Here's how the part is built. I have some questions about the finished solid (model axes, mm). Face numbers are marked on the shaded views. A direction names the side the tool comes from. Round coordinates to 2 decimals unless told otherwise and drop trailing zeros. Loops run counter-clockwise (first coordinate to the right, second up) from the corner with the lowest first, then second, coordinate; pieces in that order, holes last. Notation, with made-up numbers: M 82,39 L 98,39 A23 ccw 98,52 Z; hole C -35.75,-23.5 d9. An arc over 180 degrees is marked long. Answer as CSV lines item,"result".
```python
from build123d import *

# Parameters (mm, degrees)
SKETCH1_R           = 1
SKETCH1_R_2         = 0.5
SKETCH1_R_3         = 1.75
BOSS_EXTRUDE1_DEPTH = 2
FILLET1_R           = 2


with BuildPart() as part:
    # Sketch1 → Boss-Extrude1 (new body)
    with BuildSketch(Plane(origin=(0, 0, 0), x_dir=(1, 0, 0), z_dir=(0, 1, 0))):
        Polygon((-12.864326531, 1.102455199), (6.635673469, 1.102455199), (6.635673469, -10.897544801), (-12.864326531, -10.897544801), (-12.864326531, -4.397544801), (-21.064326531, -4.397544801), (-21.064326531, 1.102455199), align=None)
        with Locations(Location((-9.864326531, -1.897544801, 0), (0, 0, 270))):
            Circle(SKETCH1_R, mode=Mode.SUBTRACT)
        with Locations(Location((3.635673469, -1.897544801, 0), (0, 0, 270))):
            Circle(SKETCH1_R, mode=Mode.SUBTRACT)
        with Locations(Location((-11.764326531, -8.897544801, 0), (0, 0, 270))):
            Circle(SKETCH1_R_2, mode=Mode.SUBTRACT)
        with Locations(Location((-1.764326531, -8.897544801, 0), (0, 0, 270))):
            Circle(SKETCH1_R_2, mode=Mode.SUBTRACT)
        with Locations(Location((-18.064326531, -1.397544801, 0), (0, 0, 270))):
            Circle(SKETCH1_R_3, mode=Mode.SUBTRACT)
    extrude(amount=BOSS_EXTRUDE1_DEPTH)

    # Fillet1
    fillet1_edges = [part.edges().sort_by_distance(p)[0] for p in [
        (6.635673469, 1, -1.102455199),
        (6.635673469, 1, 10.897544801),
        (-12.864326531, 1, 10.897544801),
        (-12.864326531, 1, 4.397544801),
        (-21.064326531, 1, 4.397544801),
        (-21.064326531, 1, -1.102455199),
    ]]
    fillet(fillet1_edges, radius=FILLET1_R)


solid = part.part
```
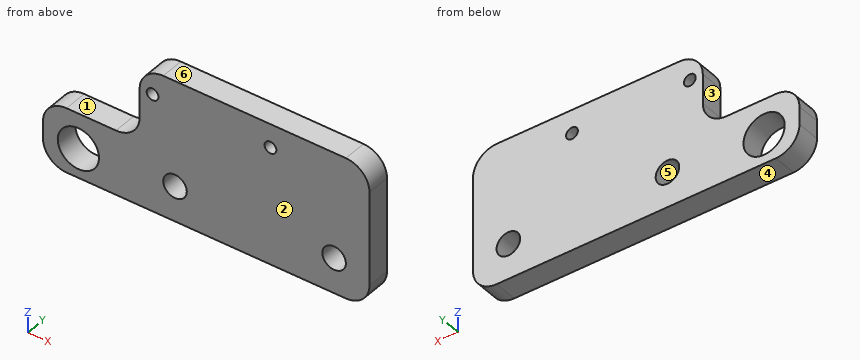
1. For P1, Ø0.6, axis at x = -16.5, y = 1, coming from the +Z side; P2, Ø1.6, axis at x = -9.86, z = 1.9, coming from the +Y side; P3, Ø1, axis at y = 1, z = 8, coming from the -X side, each with a flat end and sliding along its axis, tell me the tip position at first contact or that it passes through.
Evaluation:
P1,"stops at z = 4.4"
P2,"passes through"
P3,"stops at x = -12.86"
2. Which directions (+Z, -Z, +X, -X, +Y, -Y) give clear straight access to the entire face, cutting with the end or side of a thin tool? Please do the marked faces 1 and 2.
Evaluation:
face 1,"+Z, -X, +Y, -Y"
face 2,"+Z, -Z, +X, -X, -Y"
3. I want a section at B-B, the plane x = -18.75. Please give me the cut outline in (y, z).
Evaluation:
outline,"M 0,-1.1 L 2,-1.1 L 2,-0.21 L 0,-0.21 Z; M 0,3.01 L 2,3.01 L 2,4.4 L 0,4.4 Z"
4. If I drill on line 1 (X direction, y = 1.1, z = 8.75); line 2 (X direction, y = 0.25, z = 2.25); line 3 (X direction, y = 0.85, z = 2.5), over which ranges is the centre line in solid material (lowest first)? Write a range as [from, to].
Evaluation:
line 1,"x = [-12.86, -12.24], [-11.29, -2.24], [-1.29, 6.64]"
line 2,"x = [-21.06, -19.59], [-16.54, -10.8], [-8.93, 2.7], [4.57, 6.64]"
line 3,"x = [-21.06, -19.42], [-16.71, -10.66], [-9.07, 2.84], [4.43, 6.64]"
5. We'd pull the mould along Z, two halves only. Please class the marked faces 3, 4, 5 and 6: pulls with the +Z half, pulls with the -Z half, needs draft (parallel to the pull), parting line crosses it, or undercut.
Evaluation:
face 3,"needs draft"
face 4,"pulls with the -Z half"
face 5,"undercut"
face 6,"pulls with the +Z half"
6. I want a section at A-A, the plane y = 1.5. Please give me the cut outline in (x, z), and give its area (3 significant figures).
Evaluation:
outline,"M -21.06,0.9 A2 ccw -19.06,-1.1 L 4.64,-1.1 A2 ccw 6.64,0.9 L 6.64,8.9 A2 ccw 4.64,10.9 L -10.86,10.9 A2 ccw -12.86,8.9 L -12.86,6.4 A2 cw -14.86,4.4 L -19.06,4.4 A2 ccw -21.06,2.4 Z; hole C -18.06,1.4 d3.5; hole C -11.76,8.9 d1; hole C -9.86,1.9 d2; hole C -1.76,8.9 d1; hole C 3.64,1.9 d2"
area,"258 mm²"
7. I want a section at D-D, the plane z = 1.75. Please give me the cut outline in (x, y).
Evaluation:
outline,"M -21.06,0 L -19.78,0 L -19.78,2 L -21.06,2 Z; M -16.35,0 L -10.85,0 L -10.85,2 L -16.35,2 Z; M -8.88,0 L 2.65,0 L 2.65,2 L -8.88,2 Z; M 4.62,0 L 6.64,0 L 6.64,2 L 4.62,2 Z"
8. I want a section at C-C, the plane z = 0. Please give me the cut outline in (x, y), and give its area (3 significant figures).
Evaluation:
outline,"M -20.85,0 L -19.12,0 L -19.12,2 L -20.85,2 Z; M -17.01,0 L 6.42,0 L 6.42,2 L -17.01,2 Z"
area,"50.3 mm²"
